```python
from build123d import *

# Parameters (mm, degrees)
SKIZZE3_W                       = 2.03
SKIZZE3_H                       = 2.5
AUFSATZ_LINEAR_AUSTRAGEN1_DEPTH = 18.902
SKIZZE3_3_W                     = 2.03
SKIZZE3_3_H                     = 2.5
SCHNITT_LINEAR_AUSTRAGEN3_DEPTH = 16.402
SKIZZE2_W                       = 11
SKIZZE2_H                       = 6.3
SCHNITT_LINEAR_AUSTRAGEN4_DEPTH = 23


with BuildPart() as part:
    # Skizze1 → Rotation2 (revolve)
    with BuildSketch(Plane(origin=(0, 0, 0), x_dir=(1, 0, 0), z_dir=(0, 1, 0)), mode=Mode.PRIVATE) as rotation2_sk:
        Polygon((0.00340061, -8.034840547), (0.00340061, -10.034840547), (20.90540061, -10.034840547), (20.90540061, 5.265159453), (18.90540061, 5.265159453), (18.90540061, -2.034840547), (17.40540061, -2.034840547), (17.40540061, -4.034840547), (18.90540061, -4.034840547), (18.90540061, -8.034840547), align=None)
    revolve(rotation2_sk.sketch.rotate(Axis((0.00340061, 0, 8.034840547), (0, 0, 1)), 180), axis=Axis((0.00340061, 0, 8.034840547), (0, 0, 1)))

    # Skizze3 → Aufsatz-Linear austragen1 (add)
    with BuildSketch(Plane(origin=(0, 0, 0), x_dir=(0, 0, -1), z_dir=(1, 0, 0))):
        with Locations((-1.015, 0)):
            Rectangle(SKIZZE3_W, SKIZZE3_H)
    extrude(amount=-AUFSATZ_LINEAR_AUSTRAGEN1_DEPTH)

    # Skizze3_3 → Schnitt-Linear austragen3 (cut)
    with BuildSketch(Plane(origin=(0, 0, 0), x_dir=(0, 0, -1), z_dir=(1, 0, 0))):
        with Locations((-1.015, 0)):
            Rectangle(SKIZZE3_3_W, SKIZZE3_3_H)
    extrude(amount=-SCHNITT_LINEAR_AUSTRAGEN3_DEPTH, mode=Mode.SUBTRACT)

    # Skizze2 → Schnitt-Linear austragen4 (cut)
    with BuildSketch(Plane(origin=(0, 0, 0), x_dir=(1, 0, 0), z_dir=(0, 1, 0))):
        with Locations((0.00340061, 2.115159453)):
            Rectangle(SKIZZE2_W, SKIZZE2_H)
    extrude(amount=SCHNITT_LINEAR_AUSTRAGEN4_DEPTH, mode=Mode.SUBTRACT)


solid = part.part
```
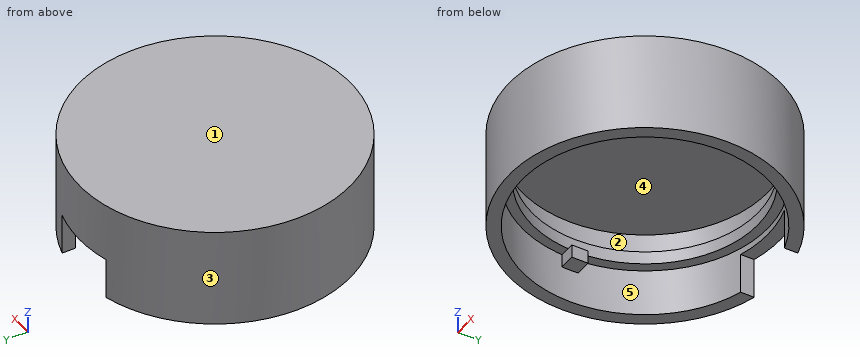
Build history of the part. All positions in model axes, mm. Face numbers are marked on the shaded views. A direction names the side the tool comes from. Give positions to 0.01 mm unless a question says otherwise; leave off trailing zeros. Order: outer loops, then holes, each group sorted by start corner. A loop starts at its lowest first (then second) coordinate and runs counter-clockwise, first axis right, second up. Notation, with made-up numbers: M -21.75,38.25 L 33.25,38.25 A17 ccw 33.25,58.25 Z; hole C 31,41 d11. An arc over 180 degrees is marked long. Return JSON: item names as keys, results as strings.
Q1. Wall check: probe 1 along Z at (x, y) = (-17, -5); probe 2 along Z at (x, y) = (12, 2); probe 3 along X at (y, z) = (-14, -3.25). Give the ranges that are in metal, low to high. Write a range as from..to.
Answer list:
{"probe 1": "z = 2.03..4.03, 8.03..10.03", "probe 2": "z = 8.03..10.03", "probe 3": "x = -15.52..-12.7, 12.7..15.52"}
Q2. Band-saw the part on C-C (z = 8.75). Give the cut face in (x, y).
Answer list:
{"outline": "C 0,0 d41.8"}
Q3. 3-axis set-ups, long thin cutter, end or side, ignore diameter. For the marked faces 3, 4 and 5: which of +Z, -Z, +X, -X, +Y, -Y reach the whole face in a straight line?
Answer list:
{"face 3": "+Z, -Z", "face 4": "none", "face 5": "-Z"}
Q4. Two-plate mould, pull along Z, no slides. Class the marked faces 1 and 2: pulls with the +Z half, pulls with the -Z half, needs draft (parallel to the pull), parting line crosses it, or undercut.
Answer list:
{"face 1": "pulls with the +Z half", "face 2": "undercut"}
Q5. Band-saw the part on D-D (x = 3). Give the cut face in (y, z), then the cut area to 3 significant figures.
Answer list:
{"outline": "M -20.69,-5.27 L -18.66,-5.27 L -18.66,2.03 L -17.14,2.03 L -17.14,4.03 L -18.66,4.03 L -18.66,8.03 L 18.66,8.03 L 18.66,4.03 L 17.14,4.03 L 17.14,2.03 L 18.66,2.03 L 18.66,1.03 L 20.69,1.03 L 20.69,10.03 L -20.69,10.03 Z", "area": "130 mm^2"}
Q6. Flat gauge pins, fed straight in: pin 1 (0.8 mm diameter, centred on x = 0, y = 19, fed in from -Z); pin 2 (1.5 mm diameter, centred on x = 3.5, z = 8, fed in from -Y); pin 3 (8 mm diameter, centred on x = 10.5, z = 0.5, fed in from -Y). Where does each tip first touch, or does it go through?
Answer list:
{"pin 1": "stops at z = 1.03", "pin 2": "stops at y = -20.72", "pin 3": "stops at y = -19.87"}
Q7. Band-saw the part on B-B (z = 6.25). Give the cut face in (x, y), then the cut area to 3 significant figures.
Answer list:
{"outline": "C 0,0 d41.8; hole C 0,0 d37.8", "area": "250 mm^2"}
